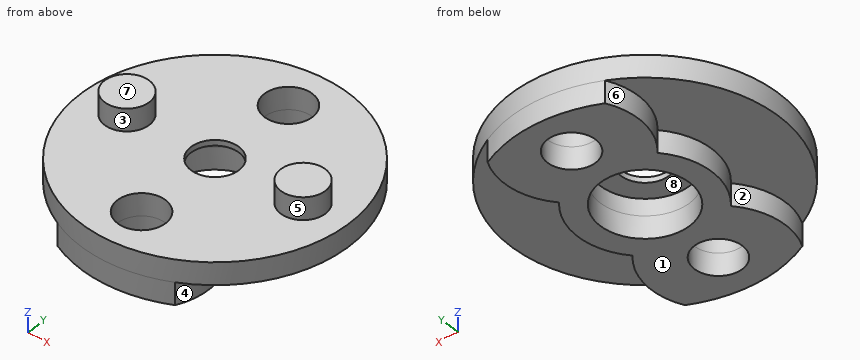
```python
from build123d import *
from build123d.topology import SkipClean

# Parameters (mm, degrees)
SKETCH1_R                  = 12
BOSS_EXTRUDE1_DEPTH        = 2
SKETCH2_R                  = 2
BOSS_EXTRUDE2_DEPTH        = 2
F_4_3_4_3_DIAMETER_HOLE1_D = 4.3
BOSS_EXTRUDE3_START        = 2
SKETCH5_R                  = 2.15
SKETCH5_R_2                = 4
BOSS_EXTRUDE3_DEPTH        = 2
SKETCH6_R                  = 4
CUT_EXTRUDE1_DEPTH         = 1.5


with BuildPart() as part:
    # Sketch1 → Boss-Extrude1 (new body)
    with BuildSketch(Plane.XY):
        Circle(SKETCH1_R)
    extrude(amount=BOSS_EXTRUDE1_DEPTH)

    # Sketch2 → Boss-Extrude2 (add)
    with BuildSketch(Plane.XY.offset(2)):
        with Locations((-8, 0)):
            Circle(SKETCH2_R)
        with Locations((8, 0)):
            Circle(SKETCH2_R)
    extrude(amount=BOSS_EXTRUDE2_DEPTH)

    # Ø4.3 (4.3) Diameter Hole1 (through all)
    with Locations(Plane.XY.offset(2)):
        with Locations((0, 8), (0, 0), (0, -8)):
            Hole(F_4_3_4_3_DIAMETER_HOLE1_D / 2)

    # Sketch5 → Boss-Extrude3 (add)
    with SkipClean():  # the faces are left unmerged after this step: merging them gives an invalid solid
        with BuildSketch(Plane(origin=(0, 0, 0), x_dir=(-1, 0, 0), z_dir=(0, 0, -1)).offset(BOSS_EXTRUDE3_START)):
            with BuildLine():
                ThreePointArc((4.472135955, -4), (6, 0), (4.472135955, 4))
                ThreePointArc((4.472135955, 4), (5.951826612, 7.241211504), (5.332682252, 10.75))
                ThreePointArc((5.332682252, 10.75), (0, 12), (-5.332682252, 10.75))
                ThreePointArc((-5.332682252, 10.75), (-5.951826612, 7.241211504), (-4.472135955, 4))
                ThreePointArc((-4.472135955, 4), (-6, 0), (-4.472135955, -4))
                ThreePointArc((-4.472135955, -4), (-5.951826612, -7.241211504), (-5.332682252, -10.75))
                ThreePointArc((-5.332682252, -10.75), (0, -12), (5.332682252, -10.75))
                ThreePointArc((5.332682252, -10.75), (5.951826612, -7.241211504), (4.472135955, -4))
            make_face()
            with Locations(Location((0, 8, 0), (0, 0, 180))):
                Circle(SKETCH5_R, mode=Mode.SUBTRACT)
            with Locations(Location((0, -8, 0), (0, 0, 180))):
                Circle(SKETCH5_R, mode=Mode.SUBTRACT)
            Circle(SKETCH5_R_2, mode=Mode.SUBTRACT)
        extrude(amount=-BOSS_EXTRUDE3_DEPTH)

    # Sketch6 → Cut-Extrude1 (cut)
    with SkipClean():  # the faces are left unmerged after this step: merging them gives an invalid solid
        with BuildSketch(Plane(origin=(0, 0, 0), x_dir=(-1, 0, 0), z_dir=(0, 0, -1))):
            Circle(SKETCH6_R)
        extrude(amount=-CUT_EXTRUDE1_DEPTH, mode=Mode.SUBTRACT)


solid = part.part
```
Read the model definition and answer for the solid it produces. Units are mm, in the model's axes. Face numbers are marked on the shaded views. A direction names the side the tool comes from. Give positions to 0.01 mm unless a question says otherwise; leave off trailing zeros. Write each loop counter-clockwise with the first axis right and the second up, starting at its lowest first coordinate (ties: lowest second). Pieces come first, ordered by that corner, then holes. Notation, with made-up numbers: (24.5, 19.25) -> (83.5, 19.25) arc R11 cw to (83.5, 36.25) -> close; hole circle Ø3 at (-31, 23.25). An arc over 180 degrees is marked (long way). Answer as a JSON object with one key per item and string values.
1) Section B-B on z = -0.8 is taken. Write down the section's boundary in (x, y).
Findings below:
{"outline": "(-5.33, -10.75) arc R12 ccw to (5.33, -10.75) arc R6 ccw to (4.47, -4) arc R6 ccw to (4.47, 4) arc R6 ccw to (5.33, 10.75) arc R12 ccw to (-5.33, 10.75) arc R6 ccw to (-4.47, 4) arc R6 ccw to (-4.47, -4) arc R6 ccw to start; hole circle Ø8 at (0, 0); hole circle Ø4.3 at (0, -8); hole circle Ø4.3 at (0, 8)"}
2) Section C-C on x = -0.5 is taken. Write down the section's boundary in (y, z), then the cut area to 3 significant figures.
Findings below:
{"outline": "(-11.99, -2) -> (-10.09, -2) -> (-10.09, 2) -> (-11.99, 2) -> close; (-5.91, -2) -> (-3.97, -2) -> (-3.97, 1.5) -> (-2.09, 1.5) -> (-2.09, 2) -> (-5.91, 2) -> close; (2.09, 1.5) -> (3.97, 1.5) -> (3.97, -2) -> (5.91, -2) -> (5.91, 2) -> (2.09, 2) -> close; (10.09, -2) -> (11.99, -2) -> (11.99, 2) -> (10.09, 2) -> close", "area": "32.6 mm^2"}
3) Section D-D on z = 3 is taken. Write down the section's boundary in (x, y), then the cut area to 3 significant figures.
Findings below:
{"outline": "circle Ø4 at (-8, 0); circle Ø4 at (8, 0)", "area": "25.1 mm^2"}
4) Flat-ended cylindrical pins translate along their axes: pin 1 Ø7 at (x, y) = (0, 0) entering from -Z; pin 2 Ø1 at (x, y) = (1, -7.5) entering from +Z; pin 3 Ø6 at (x, y) = (-9, -4) entering from -Z; pin 4 Ø5.5 at (x, y) = (0, 8) entering from +Z. Find the tip coordinate at first contact, or state that the pin passes through.
Findings below:
{"pin 1": "stops at z = 1.5", "pin 2": "passes through", "pin 3": "stops at z = 0", "pin 4": "stops at z = 2"}
5) Section A-A on y = 0 is taken. Write down the section's boundary in (x, z).
Findings below:
{"outline": "(-12, 0) -> (-6, 0) -> (-6, -2) -> (-4, -2) -> (-4, 1.5) -> (-2.15, 1.5) -> (-2.15, 2) -> (-6, 2) -> (-6, 4) -> (-10, 4) -> (-10, 2) -> (-12, 2) -> close; (2.15, 1.5) -> (4, 1.5) -> (4, -2) -> (6, -2) -> (6, 0) -> (12, 0) -> (12, 2) -> (10, 2) -> (10, 4) -> (6, 4) -> (6, 2) -> (2.15, 2) -> close"}
6) Straight lines are drawn through the part: probe 1 along Y at (x, z) = (0, 1.75); probe 2 along Y at (x, z) = (0, 1.2); probe 3 along Z at (x, y) = (0, -2.25). For each, find the intervals that lie inside material, in ascending order. Write a range as from..to.
Findings below:
{"probe 1": "y = -12..-10.15, -5.85..-2.15, 2.15..5.85, 10.15..12", "probe 2": "y = -12..-10.15, -5.85..-4, 4..5.85, 10.15..12", "probe 3": "z = 1.5..2"}
7) For a pull along Y with two mould halves and no side action, classify the marked faces 1, 2 and 3 as pulls with the +Y half, pulls with the -Y half, needs draft (parallel to the pull), parting line crosses it, or undercut.
Findings below:
{"face 1": "needs draft", "face 2": "undercut", "face 3": "parting line crosses it"}
8) A tool of negligible diameter and unlimited length cuts with its end or side. For the marked faces 4, 5, 6, 7 and 8, from which of +Z, -Z, +X, -X, +Y, -Y can it reach the whole face along a straight path? Write none if from no direction.
Findings below:
{"face 4": "-Z, +X", "face 5": "+Z", "face 6": "-Z, -X", "face 7": "+Z, +X, -X, +Y, -Y", "face 8": "-Z"}
